Work out the finished part from the listing and answer in its coordinate system (mm). Face numbers are marked on the shaded views. A direction names the side the tool comes from. Give positions to 0.01 mm unless a question says otherwise; leave off trailing zeros. Loops run counter-clockwise (first coordinate to the right, second up) from the corner with the lowest first, then second, coordinate; pieces in that order, holes last. Notation, with made-up numbers: (23, 4) - (71, 4) arc R23 cw to (71, 33) - close; hole circle Ø2 at (61, 71). An arc over 180 degrees is marked (long way). One line per question, with ' | ' between items.
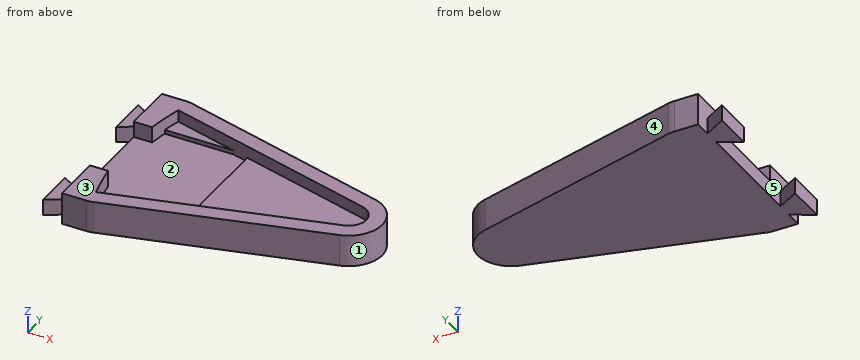
from build123d import *

# Parameters (mm, degrees)
BOSS_EXTRUDE1_DEPTH = 6
BOSS_EXTRUDE2_START = 6
BOSS_EXTRUDE2_DEPTH = 6
BOSS_EXTRUDE3_DEPTH = 6
SKETCH3_W           = 6
SKETCH3_H           = 30
CUT_EXTRUDE1_DEPTH  = 10
BOSS_EXTRUDE4_DEPTH = 1.5


with BuildPart() as part:
    # Sketch1 → Boss-Extrude1 (new body)
    # profile 1 of 2: a face of its own
    with BuildSketch(Plane.XY):
        with BuildLine():
            Line((-95.5, -34.142511157), (-86.497052813, -34.142511157))
            ThreePointArc((-86.497052813, -34.142511157), (-85.191790891, -34.05695977), (-83.908862362, -33.80176942))
            Line((-83.908862362, -33.80176942), (-3.220006135, -12.181255556))
            ThreePointArc((-3.220006135, -12.181255556), (6.127, 0), (-3.220006135, 12.181255556))
            Line((-3.220006135, 12.181255556), (-83.908862362, 33.80176942))
            ThreePointArc((-83.908862362, 33.80176942), (-85.191790891, 34.05695977), (-86.497052813, 34.142511157))
            Line((-86.497052813, 34.142511157), (-95.5, 34.142511157))
            Line((-95.5, 34.142511157), (-95.5, -34.142511157))
        make_face()
        with BuildLine():
            ThreePointArc((-4.772920406, -6.385700598), (0.127, 0), (-4.772920406, 6.385700598))
            Line((-4.772920406, 6.385700598), (-85.970442822, 28.142511157))
            ThreePointArc((-85.970442822, 28.142511157), (-89.627, 0), (-85.970442822, -28.142511157))
            Line((-85.970442822, -28.142511157), (-4.772920406, -6.385700598))
        make_face(mode=Mode.SUBTRACT)
    # profile 2 of 2: a face of its own
    with BuildSketch(Plane.XY):
        with BuildLine():
            Line((-85.970442822, -28.142511157), (-4.772920406, -6.385700598))
            ThreePointArc((-4.772920406, -6.385700598), (0.127, 0), (-4.772920406, 6.385700598))
            Line((-4.772920406, 6.385700598), (-85.970442822, 28.142511157))
            ThreePointArc((-85.970442822, 28.142511157), (-89.627, 0), (-85.970442822, -28.142511157))
        make_face()
    extrude(amount=BOSS_EXTRUDE1_DEPTH)

    # Sketch1<3> → Boss-Extrude2 (add)
    with BuildSketch(Plane.XY.offset(BOSS_EXTRUDE2_START)):
        with BuildLine():
            Line((-83.908862362, -33.80176942), (-3.220006135, -12.181255556))
            ThreePointArc((-3.220006135, -12.181255556), (6.127, 0), (-3.220006135, 12.181255556))
            Line((-3.220006135, 12.181255556), (-83.908862362, 33.80176942))
            ThreePointArc((-83.908862362, 33.80176942), (-85.191790891, 34.05695977), (-86.497052813, 34.142511157))
            Line((-86.497052813, 34.142511157), (-95.5, 34.142511157))
            Line((-95.5, 34.142511157), (-95.5, -34.142511157))
            Line((-95.5, -34.142511157), (-86.497052813, -34.142511157))
            ThreePointArc((-86.497052813, -34.142511157), (-85.191790891, -34.05695977), (-83.908862362, -33.80176942))
        make_face()
        with BuildLine():
            Line((-85.970442822, -28.142511157), (-4.772920406, -6.385700598))
            ThreePointArc((-4.772920406, -6.385700598), (0.127, 0), (-4.772920406, 6.385700598))
            Line((-4.772920406, 6.385700598), (-85.970442822, 28.142511157))
            ThreePointArc((-85.970442822, 28.142511157), (-89.627, 0), (-85.970442822, -28.142511157))
        make_face(mode=Mode.SUBTRACT)
    extrude(amount=BOSS_EXTRUDE2_DEPTH)

    # Sketch2 → Boss-Extrude3 (add)
    with BuildSketch(Plane.XY):
        Polygon((-95.5, 27.881197846), (-103.5, 32.5), (-103.5, 17.5), (-95.5, 22.118802154), align=None)
        Polygon((-103.5, -17.5), (-95.5, -22.118802154), (-95.5, -27.881197846), (-103.5, -32.5), align=None)
    extrude(amount=BOSS_EXTRUDE3_DEPTH)

    # Sketch3 → Cut-Extrude1 (cut)
    with BuildSketch(Plane.ZY.offset(95.5)):
        with Locations((9, 0)):
            Rectangle(SKETCH3_W, SKETCH3_H)
    extrude(amount=-CUT_EXTRUDE1_DEPTH, mode=Mode.SUBTRACT)

    # Sketch4 → Boss-Extrude4 (add)
    with BuildSketch(Plane.XY.offset(6)):
        with BuildLine():
            Line((-55.582177484, 20), (-55.582177484, -20))
            Line((-55.582177484, -20), (-4.772920406, -6.385700598))
            ThreePointArc((-4.772920406, -6.385700598), (0.127, 0), (-4.772920406, 6.385700598))
            Line((-4.772920406, 6.385700598), (-55.582177484, 20))
        make_face()
        with BuildLine():
            Line((-87.485682099, 21.611307008), (-61.595657104, 21.611307008))
            Line((-61.595657104, 21.611307008), (-85.970442822, 28.142511157))
            ThreePointArc((-85.970442822, 28.142511157), (-86.777777456, 24.888442961), (-87.485682099, 21.611307008))
        make_face()
        with BuildLine():
            Line((-85.970442822, -28.142511157), (-61.595657104, -21.611307008))
            Line((-61.595657104, -21.611307008), (-87.485682099, -21.611307008))
            ThreePointArc((-87.485682099, -21.611307008), (-86.777777456, -24.888442961), (-85.970442822, -28.142511157))
        make_face()
    extrude(amount=BOSS_EXTRUDE4_DEPTH)


solid = part.part
1. Find section D-D on y = 24. Write down the section's boundary in (x, z), then the cut area to 3 significant figures.
Evaluation:
outline: (-103.5, 0) - (-47.33, 0) - (-47.33, 12) - (-70.51, 12) - (-70.51, 7.5) - (-86.98, 7.5) - (-86.98, 12) - (-95.5, 12) - (-95.5, 6) - (-103.5, 6) - close | area: 552 mm2
2. Find section B-B on y = -2.5. Write down the section's boundary in (x, z), then the cut area to 3 significant figures.
Evaluation:
outline: (-95.5, 0) - (5.88, 0) - (5.88, 12) - (-0.36, 12) - (-0.36, 7.5) - (-55.58, 7.5) - (-55.58, 6) - (-95.5, 6) - close | area: 729 mm2
3. Find section A-A on z = 2.75. Write down the section's boundary in (x, y).
Evaluation:
outline: (-103.5, -32.5) - (-95.5, -27.88) - (-95.5, -34.14) - (-86.5, -34.14) arc R10 ccw to (-83.91, -33.8) - (-3.22, -12.18) arc R12.61 ccw to (-3.22, 12.18) - (-83.91, 33.8) arc R10 ccw to (-86.5, 34.14) - (-95.5, 34.14) - (-95.5, 27.88) - (-103.5, 32.5) - (-103.5, 17.5) - (-95.5, 22.12) - (-95.5, -22.12) - (-103.5, -17.5) - close
4. Consider L1, parallel to Z at x = -62, y = 18; L2, parallel to Y at x = -43.5, z = 10; L3, parallel to Z at x = -50.5, y = 11. Determine where each line is inside the solid, lowest interval first.
Evaluation:
L1: 0 to 6 | L2: -22.97 to -16.76, 16.76 to 22.97 | L3: 0 to 7.5
5. Flat-ended cylindrical pins translate along their axes: pin 1 (10 mm diameter, centred on x = -46, y = 2.5, fed in from -Z); pin 2 (5 mm diameter, centred on y = 16.5, z = 8.5, fed in from -X); pin 3 (4 mm diameter, centred on x = -99.5, y = 23.5, fed in from +Z); pin 4 (1.6 mm diameter, centred on x = -71, z = 7, fed in from +Y). Find the tip coordinate at first contact, or state that the pin passes through.
Evaluation:
pin 1: z = 0 | pin 2: x = -95.5 | pin 3: z = 6 | pin 4: y = 30.56
6. Find section C-C on z = 9.5. Write down the section's boundary in (x, y), then the cut area to 3 significant figures.
Evaluation:
outline: (-95.5, -34.14) - (-86.5, -34.14) arc R10 ccw to (-83.91, -33.8) - (-3.22, -12.18) arc R12.61 ccw to (-3.22, 12.18) - (-83.91, 33.8) arc R10 ccw to (-86.5, 34.14) - (-95.5, 34.14) - (-95.5, 15) - (-88.6, 15) arc R110.13 cw to (-85.97, 28.14) - (-4.77, 6.39) arc R6.61 cw to (-4.77, -6.39) - (-85.97, -28.14) arc R110.13 cw to (-88.6, -15) - (-95.5, -15) - close | area: 1,500 mm2
7. Which of the six approach directions +Z, -Z, +X, -X, +Y, -Y give full straight-line access (tool end or side, diameter ignored) to the marked faces 1 and 2?
Evaluation:
face 1: +Z, -Z, +X | face 2: +Z
8. Determine the mould class of the marked faces 3, 4 and 5 for opening direction X: +X half, -X half, draft (parallel to the pull), parting line (faces both ways), or undercut.
Evaluation:
face 3: draft | face 4: +X half | face 5: undercut
